Check sheet for the modelled part. Datum: model origin and axes. Units: mm. A direction names the side the tool comes from. Round coordinates to 2 decimals unless told otherwise and drop trailing zeros. Write each loop counter-clockwise with the first axis right and the second up, starting at its lowest first coordinate (ties: lowest second). Pieces come first, ordered by that corner, then holes. Notation, with made-up numbers: (-17, 22.25) -> (0, 22.25) arc R34 cw to (0, 56.25) -> close; hole circle Ø1 at (-16, 3). An arc over 180 degrees is marked (long way). Use one line per item in the form item = value. Start each with the question number.
```python
from build123d import *

# Parameters (mm, degrees)
SKETCH1_W                 = 57.15
SKETCH1_H                 = 111.125
BOSS_EXTRUDE1_DEPTH       = 9.525
SKETCH2_R                 = 6.35
CUT_EXTRUDE1_DEPTH        = 83.55
SKETCH4_W                 = 4.7625
SKETCH4_H                 = 19.05
SKETCH4_H_2               = 19.057929795
CUT_EXTRUDE2_DEPTH        = 20.05
F_4_40_TAPPED_HOLE2_D     = 2.2606
F_4_40_TAPPED_HOLE2_DEPTH = 12.7
F_4_40_TAPPED_HOLE2_TIP   = 0.679152758
SKETCH14_W                = 9.525
SKETCH14_H                = 19.05
BOSS_EXTRUDE2_DEPTH       = 19.05
HOLE1_D                   = 7.94512
HOLE1_DEPTH               = 46.0375
HOLE1_TIP                 = 2.386954861
FILLET1_R                 = 1.27
SKETCH17_W                = 53.975
SKETCH17_H                = 12.7
CUT_EXTRUDE3_DEPTH        = 20.05
F_5_40_TAPPED_HOLE1_D     = 2.5781


with BuildPart() as part:
    # Sketch1 → Boss-Extrude1 (new body, symmetric)
    with BuildSketch(Plane.XY):
        Polygon((9.525, 0), (-9.525, 0), (-9.525, 19.05), (-41.275, 19.05), (-41.275, 131.596658994), (-41.275, 152.4), (41.275, 152.4), (41.275, 131.596658994), (41.275, 19.05), (9.525, 19.05), align=None)
        with Locations((0, 84.1375)):
            Rectangle(SKETCH1_W, SKETCH1_H, mode=Mode.SUBTRACT)
    extrude(amount=BOSS_EXTRUDE1_DEPTH, both=True)

    # Sketch2 → Cut-Extrude1 (cut, through all)
    with BuildSketch(Plane.ZY.offset(41.275)):
        with Locations((0, 57.15)):
            Circle(SKETCH2_R)
        with Locations((0, 120.65)):
            Circle(SKETCH2_R)
    extrude(amount=-CUT_EXTRUDE1_DEPTH, mode=Mode.SUBTRACT)

    # Sketch4 → Cut-Extrude2 (cut, through all)
    with BuildSketch(Plane(origin=(0, 0, -9.525), x_dir=(-1, 0, 0), z_dir=(0, 0, -1))):
        with Locations((-7.14375, 9.525)):
            Rectangle(SKETCH4_W, SKETCH4_H)
        with Locations((7.14375, 9.528964897)):
            Rectangle(SKETCH4_W, SKETCH4_H_2)
    extrude(amount=-CUT_EXTRUDE2_DEPTH, mode=Mode.SUBTRACT)

    # #4-40 Tapped Hole2
    with Locations(Plane(origin=(41.275, 0, 0), x_dir=(0, 0, -1), z_dir=(1, 0, 0))):
        with Locations((0, 80.1624), (0, 34.1376)):
            Hole(F_4_40_TAPPED_HOLE2_D / 2, depth=F_4_40_TAPPED_HOLE2_DEPTH)
            with Locations((0, 0, -(F_4_40_TAPPED_HOLE2_DEPTH + F_4_40_TAPPED_HOLE2_TIP / 2))):  # 118° drill point
                Cone(0, F_4_40_TAPPED_HOLE2_D / 2, F_4_40_TAPPED_HOLE2_TIP, mode=Mode.SUBTRACT)

    # Sketch14 → Boss-Extrude2 (add)
    with BuildSketch(Plane.XZ):
        Rectangle(SKETCH14_W, SKETCH14_H)
    extrude(amount=BOSS_EXTRUDE2_DEPTH)

    # Hole1
    with Locations(Plane.ZY.offset(4.7625)):
        with Locations((0, 6.35), (0, -8.89)):
            Hole(HOLE1_D / 2, depth=HOLE1_DEPTH)
            with Locations((0, 0, -(HOLE1_DEPTH + HOLE1_TIP / 2))):  # 118° drill point
                Cone(0, HOLE1_D / 2, HOLE1_TIP, mode=Mode.SUBTRACT)

    # Fillet1
    fillet1_edges = [part.edges().sort_by_distance(p)[0] for p in [
        (28.575, 139.7, 0),
        (-28.575, 139.7, 0),
        (-28.575, 28.575, 0),
        (28.575, 28.575, 0),
        (-4.7625, 19.057929795, 0),
        (4.7625, 19.05, 0),
    ]]
    fillet(fillet1_edges, radius=FILLET1_R)

    # Sketch17 → Cut-Extrude3 (cut, through all)
    with BuildSketch(Plane.XY.offset(9.525)):
        with Locations((0, 146.05)):
            Rectangle(SKETCH17_W, SKETCH17_H)
    extrude(amount=-CUT_EXTRUDE3_DEPTH, mode=Mode.SUBTRACT)

    # #5-40 Tapped Hole1 (through all)
    with Locations(Plane(origin=(0, 0, 9.525), x_dir=(-1, 0, 0), z_dir=(0, 0, 1))):
        with Locations((-34.13125, -133.35), (34.13125, -133.35)):
            Hole(F_5_40_TAPPED_HOLE1_D / 2)


solid = part.part
```
1. Mould release check, pull along Y, two halves, no side actions. Record for faces 5 (the face through (28.575, 83, 0)), 6 (the face through (-35.014, 126.946, -0.827)), 7 (the face through (0, -19.05, 0)), 8 (the face through (-41.275, 87, 0)): +Y half, -Y half, draft (parallel to the pull), parting line (faces both ways), or undercut.
2. Depth check by flat-ended pin: pin 1 (2 mm diameter, centred on x = 16.5, z = -3, fed in from +Y) (3 decimals); pin 2 (5.5 mm diameter, centred on x = 30, z = 4, fed in from -Y); pin 3 (2 mm diameter, centred on y = 80.16, z = 0, fed in from +X) (3 decimals); pin 4 (3 mm diameter, centred on x = 34.13, y = 133.35, fed in from +Z) (3 decimals). Enter the tip coordinate at first touch or a pass-through.
3. Sectioned sample at C-C (x = 13.5). Enter the section's corners in (y, z) (3 decimals), and give its area (3 significant figures).
4. Sectioned sample at D-D (y = 6.35). Enter the section's corners in (x, z) (1 decimal), and give its area (3 significant figures).
5. Scan lines: probe 1 along Y at (x, z) = (38.5, 0); probe 2 along X at (y, z) = (47, 0.5) (3 decimals); probe 3 along Z at (x, y) = (-34, 57) (3 decimals). Record each from-to range of solid material in increasing order.
6. Sectioned sample at B-B (y = 90.5). Enter the section's corners in (x, z) (3 decimals), and give its area (3 significant figures).
7. Sectioned sample at A-A (y = 57.15). Enter the section's corners in (x, z) (3 decimals), and give its area (3 significant figures).
8. Tool access check on faces 1 (the face through (4.762, 0, 0)), 2 (the face through (-28.575, 83, 0)), 3 (the face through (-26.988, 146, 0)), 4 (the face through (-8, 19.058, 0)). Record the directions out of +Z, -Z, +X, -X, +Y, -Y that give a thin tool (end or side, any length) a straight path to the whole face; none if there is none.
Returned:
q1.face_5 = undercut
q1.face_6 = undercut
q1.face_7 = -Y half
q1.face_8 = draft
q2.pin_1 = 28.575
q2.pin_2 = 19.05
q2.pin_3 = -28.575
q2.pin_4 = 9.525
q3.outline = (19.05, -9.525) -> (28.575, -9.525) -> (28.575, 9.525) -> (19.05, 9.525) -> close
q3.area = 181 mm^2
q4.outline = (-4.8, -9.5) -> (4.8, -9.5) -> (4.8, -4) -> (-4.8, -4) -> close; (-4.8, 4) -> (4.8, 4) -> (4.8, 9.5) -> (-4.8, 9.5) -> close
q4.area = 106 mm^2
q5.probe_1 = 19.05 to 33.01, 35.27 to 50.8, 63.5 to 79.03, 81.29 to 114.3, 127 to 152.4
q5.probe_2 = -41.275 to -28.575, 28.575 to 41.275
q5.probe_3 = -9.525 to -6.348, 6.348 to 9.525
q6.outline = (-41.275, -9.525) -> (-28.575, -9.525) -> (-28.575, 9.525) -> (-41.275, 9.525) -> close; (28.575, -9.525) -> (41.275, -9.525) -> (41.275, 9.525) -> (28.575, 9.525) -> close
q6.area = 484 mm^2
q7.outline = (-41.275, -9.525) -> (-28.575, -9.525) -> (-28.575, -6.35) -> (-41.275, -6.35) -> close; (-41.275, 6.35) -> (-28.575, 6.35) -> (-28.575, 9.525) -> (-41.275, 9.525) -> close; (28.575, -9.525) -> (41.275, -9.525) -> (41.275, -6.35) -> (28.575, -6.35) -> close; (28.575, 6.35) -> (41.275, 6.35) -> (41.275, 9.525) -> (28.575, 9.525) -> close
q7.area = 161 mm^2
q8.face_1 = +Z, -Z, +X, -Y
q8.face_2 = +Z, -Z
q8.face_3 = +Z, -Z, +Y
q8.face_4 = +Z, -Z, -X, -Y
